Verification items for the finished model (mm, model axes). Coordinates: 2 decimals unless noted, no trailing zeros. Order: outer loops, then holes, each group sorted by start corner. A loop starts at its lowest first (then second) coordinate and runs counter-clockwise, first axis right, second up. Notation, with made-up numbers: M 13.5,-21 L 32.5,-21 A32 cw 32.5,5 Z; hole C 32,54 d9. An arc over 180 degrees is marked long. Return JSON: item names as keys, results as strings. Group by question number.
1. Section check D-D, the plane x = 216. Record the cut outline in (y, z).
2. Section check A-A, the plane x = 100. Record the cut outline in (y, z), plus the area to 3 significant figures.
3. Gauge pin test, flat ends, axial feed: pin 1 (3 mm diameter, centred on y = 13, z = 2.5, fed in from -X); pin 2 (3 mm diameter, centred on y = 7, z = 3.5, fed in from +X); pin 3 (1.5 mm diameter, centred on x = 191.5, z = 1.5, fed in from -Y). Record the tip position at first contact, or that the pin passes through.
4. Section check C-C, the plane z = 2.55. Give the number of separate pieces and of enclosed holes in the cut face, plus the area to 3 significant figures.
5. Material ranges on line 1 along X through (y, z) = (6.5, 2.45); line 2 along Y through (x, z) = (100, 1.9); line 3 along Y through (x, z) = (117, 2.55), recorded low to high.
6. Section check B-B, the plane y = 25. Record the cut outline in (x, z), plus the area to 3 significant figures.
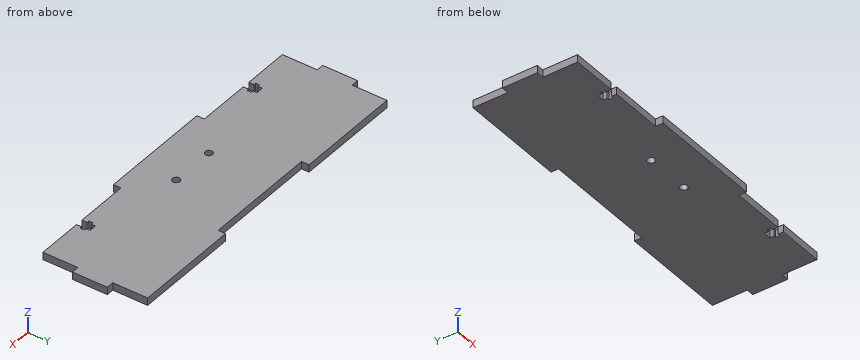
```python
from build123d import *

# Parameters (mm, degrees)
SALIENTE_EXTRUIR1_DEPTH = 5
CORTAR_EXTRUIR1_DEPTH   = 5
CROQUIS3_W              = 76.666666666
CROQUIS3_H              = 5
CORTAR_EXTRUIR2_DEPTH   = 10
CROQUIS4_R              = 2.5
CORTAR_EXTRUIR3_DEPTH   = 10


with BuildPart() as part:
    # Croquis1 → Saliente-Extruir1 (new body)
    with BuildSketch(Plane.XY):
        Polygon((76.666666667, 5), (76.666666667, 0), (153.333333333, 0), (153.333333333, 5), (225, 5), (225, 28.333333333), (230, 28.333333333), (230, 51.666666667), (225, 51.666666667), (225, 75), (5, 75), (5, 51.666666667), (0, 51.666666667), (0, 28.333333333), (5, 28.333333333), (5, 5), align=None)
    extrude(amount=SALIENTE_EXTRUIR1_DEPTH)

    # Croquis2 → Cortar-Extruir1 (cut)
    with BuildSketch(Plane.XY.offset(5)):
        Polygon((35.833333333, 5), (35.833333333, 8.5), (34.333333333, 8.5), (34.333333333, 11.3), (35.833333333, 11.3), (35.833333333, 14), (40.833333333, 14), (40.833333333, 11.3), (42.333333333, 11.3), (42.333333333, 8.5), (40.833333333, 8.5), (40.833333333, 5), align=None)
        Polygon((189.166666667, 5), (189.166666667, 8.5), (187.666666667, 8.5), (187.666666667, 11.3), (189.166666667, 11.3), (189.166666667, 14), (194.166666667, 14), (194.166666667, 11.3), (195.666666667, 11.3), (195.666666667, 8.5), (194.166666667, 8.5), (194.166666667, 5), align=None)
    extrude(amount=-CORTAR_EXTRUIR1_DEPTH, mode=Mode.SUBTRACT)

    # Croquis3 → Cortar-Extruir2 (cut)
    with BuildSketch(Plane.XY.offset(5)):
        with Locations((115, 72.5)):
            Rectangle(CROQUIS3_W, CROQUIS3_H)
    extrude(amount=-CORTAR_EXTRUIR2_DEPTH, mode=Mode.SUBTRACT)

    # Croquis4 → Cortar-Extruir3 (cut)
    with BuildSketch(Plane.XY.offset(5)):
        with Locations((100, 25)):
            Circle(CROQUIS4_R)
        with Locations((130, 25)):
            Circle(CROQUIS4_R)
    extrude(amount=-CORTAR_EXTRUIR3_DEPTH, mode=Mode.SUBTRACT)


solid = part.part
```
Answers follow:
{
 "1": {"outline": "M 5,0 L 75,0 L 75,5 L 5,5 Z"},
 "2": {"outline": "M 0,0 L 22.5,0 L 22.5,5 L 0,5 Z; M 27.5,0 L 70,0 L 70,5 L 27.5,5 Z", "area": "325 mm^2"},
 "3": {"pin 1": "x = 5", "pin 2": "x = 225", "pin 3": "y = 14"},
 "4": {"separate pieces": "1", "enclosed holes": "2", "area": "15,500 mm^2"},
 "5": {"line 1": "5 to 35.83, 40.83 to 189.17, 194.17 to 225", "line 2": "0 to 22.5, 27.5 to 70", "line 3": "0 to 70"},
 "6": {"outline": "M 5,0 L 97.5,0 L 97.5,5 L 5,5 Z; M 102.5,0 L 127.5,0 L 127.5,5 L 102.5,5 Z; M 132.5,0 L 225,0 L 225,5 L 132.5,5 Z", "area": "1,050 mm^2"}
}
